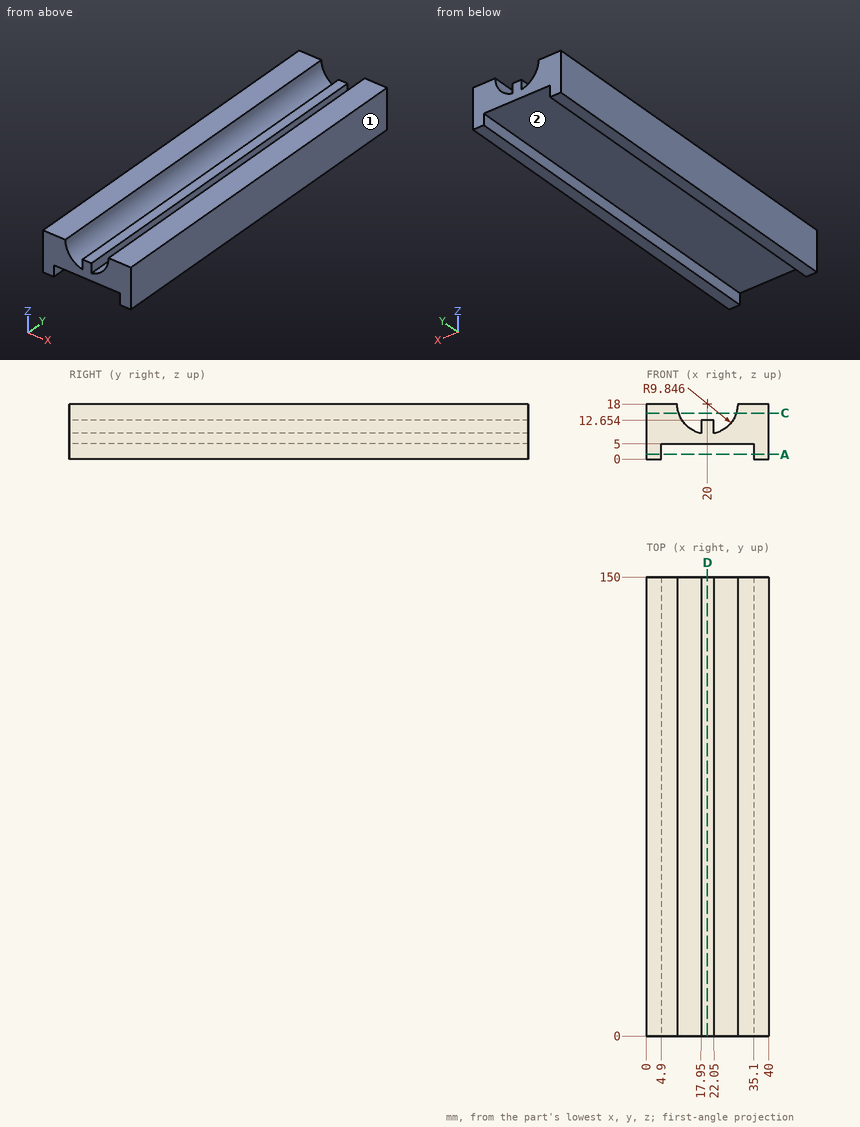
Answer from the drawing. Dimensions are ordinates in mm from the lowest x, y and z of the part. A direction names the side the tool comes from. Coordinates: 2 decimals unless noted, no trailing zeros. Loops run counter-clockwise (first coordinate to the right, second up) from the corner with the lowest first, then second, coordinate; pieces in that order, holes last. Notation, with made-up numbers: (15.25, 0.5) - (59.25, 0.5) arc R21 cw to (59.25, 36.5) - close; hole circle Ø8 at (68, 89.25). An arc over 180 degrees is marked (long way). Answer in a Markdown table with one row per item.
1. Find section D-D, the plane x = 20. Write down the section's boundary in (y, z), then the cut area to 3 significant figures.
Conclusion:
| item | result |
|---|---|
| outline | (0, 5) - (150, 5) - (150, 12.65) - (0, 12.65) - close |
| area | 1,150 mm² |
2. Find section A-A, the plane z = 1.5. Write down the section's boundary in (x, y), then the cut area to 3 significant figures.
Conclusion:
| item | result |
|---|---|
| outline | (0, 0) - (4.9, 0) - (4.9, 150) - (0, 150) - close; (35.1, 0) - (40, 0) - (40, 150) - (35.1, 150) - close |
| area | 1,470 mm² |
3. Find section C-C, the plane z = 15. Write down the section's boundary in (x, y), then the cut area to 3 significant figures.
Conclusion:
| item | result |
|---|---|
| outline | (0, 0) - (10.62, 0) - (10.62, 150) - (0, 150) - close; (29.38, 0) - (40, 0) - (40, 150) - (29.38, 150) - close |
| area | 3,190 mm² |
4. Given pin 1 (3.5 mm diameter, centred on x = 20.5, y = 98, fed in from +Z), flat-ended and moving along its own axis, determine where the tip first touches the part or whether it passes through.
Conclusion:
| item | result |
|---|---|
| pin 1 | stops at z = 12.65 |
5. Straight lines are drawn through the part: line 1 (X direction, y = 29, z = 1); line 2 (Z direction, x = 21, y = 88.5); line 3 (Z direction, x = 31, y = 128). For each, find the intervals that lie inside material, in ascending order.
Conclusion:
| item | result |
|---|---|
| line 1 | x = 0 to 4.9, 35.1 to 40 |
| line 2 | z = 5 to 12.65 |
| line 3 | z = 5 to 18 |
6. Which of the six approach directions +Z, -Z, +X, -X, +Y, -Y give full straight-line access (tool end or side, diameter ignored) to the marked faces 1 and 2?
Conclusion:
| item | result |
|---|---|
| face 1 | +Z, -Z, +X, +Y, -Y |
| face 2 | -Z, +Y, -Y |
